```python
from build123d import *


with BuildPart() as f1:
    # F0 (on Front) → F1 (revolve)
    with BuildSketch(Plane.XZ):
        Polygon((6.946762, 30.415747), (5.848836, 25.608581), (11.263847, 24.371827), (21.624854, 24.371827), (23.927299, 17.752293), (37.166368, 17.464489), (36.30295, 27.249882), (59.327412, 27.249882), (69.976225, 20.63035), (72.278671, 26.098661), (82.351863, 26.098661), (86.956762, 35.020638), (84.078699, 42.215787), (75.444527, 42.215787), (69.688417, 42.215787), (69.688417, 37.323084), (65.371335, 37.323084), (65.371335, 40.776756), (57.312772, 40.776756), (57.312772, 34.445029), (51.268846, 34.445029), (51.268846, 41.06456), (23.351688, 41.06456), align=None)
    revolve(axis=Axis((38.350116, 0, 0), (1, 0, 0)))


solid = f1.part
```
Check sheet for the modelled part. Datum: model origin and axes. Units: mm. A direction names the side the tool comes from. Round coordinates to 2 decimals unless told otherwise and drop trailing zeros. Loops run counter-clockwise (first coordinate to the right, second up) from the corner with the lowest first, then second, coordinate; pieces in that order, holes last. Notation, with made-up numbers: M 85.5,-34.5 L 97.5,-34.5 A23 cw 97.5,-8.5 Z; hole C 26.25,26.5 d10. An arc over 180 degrees is marked long. Answer as a JSON object with one key per item and string values.
1. Gauge pin test, flat ends, axial feed: P1, Ø2, axis at x = 73.5, z = -26.5, coming from the -Y side; P2, Ø2, axis at x = 40.5, z = 24.5, coming from the -Y side; P3, Ø6, axis at x = 50.5, y = -4.5, coming from the -Z side. Record the tip position at first contact, or that the pin passes through.
Reply:
{"P1": "stops at y = -33.64", "P2": "stops at y = -33.68", "P3": "stops at z = -41.04"}
2. Section check A-A (x = 74.5). Record the boundary of the cut face in (y, z).
Reply:
{"outline": "C 0,0 d84.43; hole C 0,0 d52.2"}
3. Scan lines: line 1 (Y direction, x = 47, z = 0); line 2 (Y direction, x = 78, z = 0); line 3 (Z direction, x = 13, y = -0.5). Record each from-to range of solid material in increasing order.
Reply:
{"line 1": "y = -41.06 to -27.25, 27.25 to 41.06", "line 2": "y = -42.22 to -26.1, 26.1 to 42.22", "line 3": "z = -34.34 to -24.37, 24.37 to 34.34"}
4. Access from +Z, -Z, +X, -X, +Y, -Y to the whole of each face (thin tool, end or side, straight path). Record for faces 4 (the cylindrical face through (16.517, -24.164, -3.173)), 5 (the cylindrical face through (77.386, 23.154, 12.043)), 6 (the flat face through (69.688, 28, 25)).
Reply:
{"face 4": "-X", "face 5": "+X", "face 6": "none"}
5. Mould release check, pull along Y, two halves, no side actions. Record for faces 1 (the flat face through (65.371, 33, -18)), 2 (the conical face through (30.64, -5.288, 16.793)), 3 (the cylindrical face through (61.286, -1.793, -40.737)): pulls with the +Y half, pulls with the -Y half, needs draft (parallel to the pull), parting line crosses it, or undercut.
Reply:
{"face 1": "needs draft", "face 2": "undercut", "face 3": "parting line crosses it"}
6. Section check B-B (x = 18.5). Record the boundary of the cut face in (y, z), plus the area to 3 significant figures.
Reply:
{"outline": "C 0,0 d75.83; hole C 0,0 d48.74", "area": "2,650 mm²"}
